Answer from the drawing. Dimensions are ordinates in mm from the lowest x, y and z of the part. A direction names the side the tool comes from. Give positions to 0.01 mm unless a question says otherwise; leave off trailing zeros. Order: outer loops, then holes, each group sorted by start corner. A loop starts at its lowest first (then second) coordinate and runs counter-clockwise, first axis right, second up. Notation, with made-up numbers: (7, -23) -> (63, -23) arc R27 ccw to (63, -1) -> close; hole circle Ø8 at (-19.5, -1). An arc over 180 degrees is marked (long way). Answer as a JSON object with one key per item and string values. Group by question number.
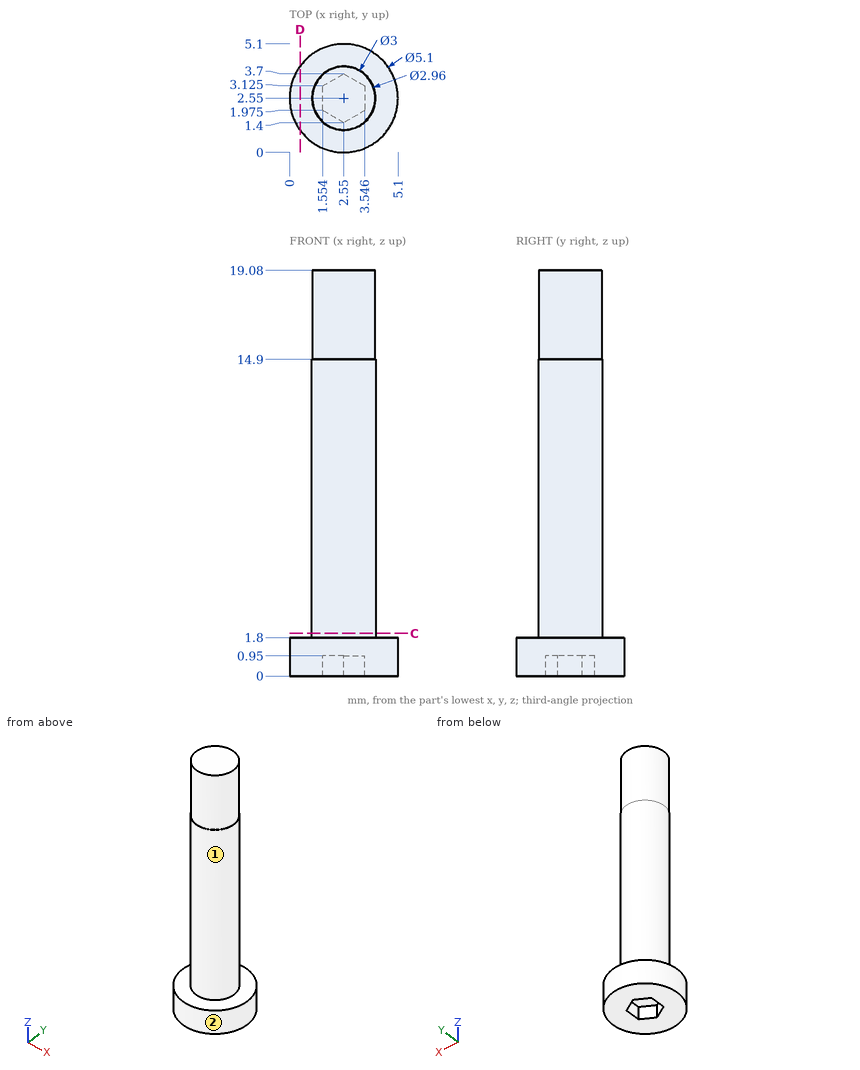
(1) Flat-ended cylindrical pins translate along their axes: pin 1 Ø3 at (x, z) = (4, 3) entering from +Y; pin 2 Ø1.5 at (y, z) = (3, 7) entering from -X; pin 3 Ø1 at (x, z) = (1, 5.5) entering from -Y. Find the tip coordinate at first contact, or state that the pin passes through.
(2) Which of the six approach directions +Z, -Z, +X, -X, +Y, -Y give full straight-line access (tool end or side, diameter ignored) to the marked faces 1 and 2?
(3) A cutting plane is placed at C-C (z = 2). Determine the outline of the cut face in (x, y), and give its area (3 significant figures).
(4) A cutting plane is placed at D-D (x = 0.5). Determine the outline of the cut face in (y, z).
(5) Find the intervals of material crossed by line 1 along Y through (x, z) = (2.6, 13.25); line 2 along Z through (x, y) = (3.3, 0.45), in increasing order. Write a range as [from, to].
Check sheet entries:
{
 "1": {"pin 1": "stops at y = 5.04", "pin 2": "stops at x = 1.05", "pin 3": "stops at y = 1.48"},
 "2": {"face 1": "+Z", "face 2": "+Z, -Z"},
 "3": {"outline": "circle Ø3 at (2.55, 2.55)", "area": "7.07 mm2"},
 "4": {"outline": "(1.03, 0) -> (4.07, 0) -> (4.07, 1.8) -> (1.03, 1.8) -> close"},
 "5": {"line 1": "y = [1.05, 4.05]", "line 2": "z = [0, 1.8]"}
}
